from build123d import *

# Parameters (mm, degrees)
F0_R     = 6
F0_R_2   = 1.1
F1_DEPTH = 2.8
F2_R     = 6
F3_DEPTH = 5.5
F5_DEPTH = 3
F6_R     = 0.5
F7_R     = 2.4
F8_DEPTH = 5


with BuildPart() as f1:
    # F0 (on Top) → F1 (new body)
    with BuildSketch(Plane.XY):
        Circle(F0_R)
        with Locations((-3.175, 0)):
            Circle(F0_R_2, mode=Mode.SUBTRACT)
        with Locations((3.175, 0)):
            Circle(F0_R_2, mode=Mode.SUBTRACT)
    extrude(amount=F1_DEPTH)

    # F2 (on face) → F3 (join)
    with BuildSketch(Plane(origin=(0, 0, 0), x_dir=(1, 0, 0), z_dir=(0, 0, -1))):
        Circle(F2_R)
    extrude(amount=F3_DEPTH)

    # F4 (on face) → F5 (cut)
    with BuildSketch(Plane.XY.offset(2.8)):
        with BuildLine():
            ThreePointArc((3.968627, 4.5), (0, 6), (-3.968627, 4.5))
            Line((-3.968627, 4.5), (-1.968627, 4.5))
            Line((-1.968627, 4.5), (-1.968627, 2.5))
            Line((-1.968627, 2.5), (1.968627, 2.5))
            Line((1.968627, 2.5), (1.968627, 4.5))
            Line((1.968627, 4.5), (3.968627, 4.5))
        make_face()
    extrude(amount=-F5_DEPTH, mode=Mode.SUBTRACT)

    # F6
    f6_edges = [f1.edges().sort_by_distance(p)[0] for p in [
        (-3.968627, 4.5, 1.3),
        (-1.968627, 4.5, 1.3),
        (1.968627, 2.5, 1.3),
        (1.968627, 4.5, 1.3),
        (3.968627, 4.5, 1.3),
        (-1.968627, 2.5, 1.3),
    ]]
    fillet(f6_edges, radius=F6_R)

    # F7 (on face) → F8 (cut)
    with BuildSketch(Plane(origin=(0, 0, -5.5), x_dir=(1, 0, 0), z_dir=(0, 0, -1))):
        Circle(F7_R)
    extrude(amount=-F8_DEPTH, mode=Mode.SUBTRACT)


solid = f1.part
Build history of the part. All positions in model axes, mm. A direction names the side the tool comes from. Round coordinates to 2 decimals unless told otherwise and drop trailing zeros. Loops run counter-clockwise (first coordinate to the right, second up) from the corner with the lowest first, then second, coordinate; pieces in that order, holes last. Notation, with made-up numbers: (-39, 28.5) -> (1, 28.5) arc R25 ccw to (1, 41.5) -> close; hole circle Ø11 at (-22.75, 4). An arc over 180 degrees is marked (long way). Use CSV: the item, a comma, the result in double quotes. Start each with the question number.
Q1. Saw through at D-D on z = -0.75. Give the cut face in (x, y), and give its area (3 significant figures).
Q2. Drill centre lines: L1, parallel to X at y = 0, z = -2.4; L2, parallel to X at y = -0.75, z = 2; L3, parallel to Z at x = 3.25, y = -0.75. Where is each one in solid material? Low to high.
Q3. Saw through at B-B on x = 0. Give the cut face in (y, z), and give its area (3 significant figures).
Q4. Which spindle directions (+Z, -Z, +X, -X, +Y, -Y) get a long thin tool onto all of the face, cutting with end or side? Do faces 4 (the face through (1.29, -2.024, -3.035)), 5 (the face through (3, 4.5, 1)), 6 (the face through (1.969, 3.5, 1.3)), 7 (the face through (0, -1, 2.8)), 8 (the face through (-2.126, 0.33, 1.38)). Say none if no direction does.
Q5. Saw through at C-C on y = -0.75. Give the cut face in (x, z), and give its area (3 significant figures).
Q6. Mould opens along X. For faces 1 (the face through (-0.78, -5.95, -1.29)), 2 (the face through (-3, 4.5, 1)), 3 (the face through (3, 0, 0)) say: +X half, -X half, draft (parallel to the pull), parting line (faces both ways), or undercut.
Q7. Saw through at A-A on z = 1.5. Give the cut face in (x, y) (3 decimals).
Q8. Flat gauge pins, fed straight in: pin 1 Ø1.1 at (x, y) = (3, 0) entering from +Z; pin 2 Ø0.8 at (y, z) = (3.5, 1) entering from -X; pin 3 Ø2.5 at (x, z) = (0.5, 2) entering from +Y. Where does each tip first touch, or does it go through?
Solutions:
1,outline,"circle Ø12 at (0, 0); hole circle Ø4.8 at (0, 0)"
1,area,"95.0 mm^2"
2,L1,"x = -6 to -2.4, 2.4 to 6"
2,L2,"x = -5.95 to -3.98, -2.37 to 2.37, 3.98 to 5.95"
2,L3,"z = -5.5 to 0"
3,outline,"(-6, -5.5) -> (-2.4, -5.5) -> (-2.4, -0.5) -> (2.4, -0.5) -> (2.4, -5.5) -> (6, -5.5) -> (6, -0.2) -> (2.5, -0.2) -> (2.5, 2.8) -> (-6, 2.8) -> close"
3,area,"65.1 mm^2"
4,face 4,"-Z"
4,face 5,"+Z, +X, -X, +Y"
4,face 6,"+Z, +Y"
4,face 7,"+Z, +X, -X, +Y, -Y"
4,face 8,"+Z"
5,outline,"(-5.95, -5.5) -> (-2.28, -5.5) -> (-2.28, -0.5) -> (2.28, -0.5) -> (2.28, -5.5) -> (5.95, -5.5) -> (5.95, 2.8) -> (3.98, 2.8) -> (3.98, 0) -> (2.37, 0) -> (2.37, 2.8) -> (-2.37, 2.8) -> (-2.37, 0) -> (-3.98, 0) -> (-3.98, 2.8) -> (-5.95, 2.8) -> close"
5,area,"67.0 mm^2"
6,face 1,"parting line"
6,face 2,"draft"
6,face 3,"undercut"
7,outline,"(-4.118, 4.364) arc R6 ccw (long way) to (4.118, 4.364) arc R0.5 ccw to (3.775, 4.5) -> (2.469, 4.5) arc R0.5 ccw to (1.969, 4) -> (1.969, 3) arc R0.5 cw to (1.469, 2.5) -> (-1.469, 2.5) arc R0.5 cw to (-1.969, 3) -> (-1.969, 4) arc R0.5 ccw to (-2.469, 4.5) -> (-3.775, 4.5) arc R0.5 ccw to start; hole circle Ø2.2 at (-3.175, 0); hole circle Ø2.2 at (3.175, 0)"
8,pin 1,"stops at z = 0"
8,pin 2,"stops at x = -5.14"
8,pin 3,"stops at y = 2.59"
